Model file for the job. Use its own axes, mm. A direction names the side the tool comes from. Round coordinates to 2 decimals unless told otherwise and drop trailing zeros. Order: outer loops, then holes, each group sorted by start corner. A loop starts at its lowest first (then second) coordinate and runs counter-clockwise, first axis right, second up. Notation, with made-up numbers: (62.5, -0.5) - (95.5, -0.5) arc R16 ccw to (95.5, 17.5) - close; hole circle Ø3 at (58, 78). An arc over 180 degrees is marked (long way). Put each result on its own line as item: value. Start each with the question number.
Item 1: Mould opens along Z. For faces 4 (the face through (0, 0, -110)), 5 (the face through (23.846, -7.509, -102.395)), 6 (the face through (-17, -17, 65)) say: pulls with the +Z half, pulls with the -Z half, needs draft (parallel to the pull), parting line crosses it, or undercut.
Item 2: Pin check, flat tips, straight feed: pin 1 Ø8 at (x, z) = (-15, -51.5) entering from -Y; pin 2 Ø2.5 at (x, y) = (0, 17.5) entering from +Z; pin 3 Ø2.5 at (x, y) = (0, -17.5) entering from -Z. Stop position of each tip, or through.
Item 3: Probe probe 1 along Y at (x, z) = (0, -102.25); probe 2 along Z at (x, y) = (20, -5.5); probe 3 along X at (y, z) = (-17, -103). List the from-to ranges inside material, lowest first.
Item 4: Which spindle directions (+Z, -Z, +X, -X, +Y, -Y) get a long thin tool onto all of the face, cutting with end or side? Do faces 1 (the face through (22.4, 7.1, -13.9)), 2 (the face through (-1.08, -4.88, 112.96)), 3 (the face through (0, 0, 116)). Say none if no direction does.
Item 5: Saw through at B-B on x = 7.5. List the corners of the cut face in (y, z).
Item 6: Saw through at A-A on z = -40.5. List the corners of the cut face in (x, y).
```python
from build123d import *

# Parameters (mm, degrees)
SKETCH1_R                 = 23.5
BOSS_EXTRUDE1_DEPTH       = 110
SKETCH2_R                 = 5
BOSS_EXTRUDE2_DEPTH       = 6
SKETCH5_R                 = 25
BOSS_EXTRUDE5_DEPTH       = 45
BOSS_EXTRUDE6_START       = -15
SKETCH6_R                 = 25
BOSS_EXTRUDE6_DEPTH       = 15
M4X0_7_TAPPED_HOLE1_D     = 3.3
M4X0_7_TAPPED_HOLE1_DEPTH = 20
M4X0_7_TAPPED_HOLE1_TIP   = 0.991420021


with BuildPart() as part:
    # Sketch1 → Boss-Extrude1 (new, symmetric)
    with BuildSketch(Plane.XY):
        Circle(SKETCH1_R)
    extrude(amount=BOSS_EXTRUDE1_DEPTH, both=True)

    # Sketch2 → Boss-Extrude2 (add)
    with BuildSketch(Plane.XY.offset(110)):
        Circle(SKETCH2_R)
    extrude(amount=BOSS_EXTRUDE2_DEPTH)

    # Sketch5 → Boss-Extrude5 (add)
    with BuildSketch(Plane.XY.offset(110)):
        Circle(SKETCH5_R)
    extrude(amount=-BOSS_EXTRUDE5_DEPTH)

    # Sketch6 → Boss-Extrude6 (add)
    with BuildSketch(Plane(origin=(0, 0, -110), x_dir=(-1, 0, 0), z_dir=(0, 0, -1)).offset(BOSS_EXTRUDE6_START)):
        with Locations(Location((0, 0, 0), (0, 0, 180))):
            Circle(SKETCH6_R)
    extrude(amount=BOSS_EXTRUDE6_DEPTH)

    # M4x0.7 Tapped Hole1
    with Locations(Plane(origin=(0, 17.5, -110), x_dir=(-1, 0, 0), z_dir=(0, 0, -1))):
        with Locations((0, 0), (17.5, -17.5), (0, -35), (-17.5, -17.5)):
            Hole(M4X0_7_TAPPED_HOLE1_D / 2, depth=M4X0_7_TAPPED_HOLE1_DEPTH)
            with Locations((0, 0, -(M4X0_7_TAPPED_HOLE1_DEPTH + M4X0_7_TAPPED_HOLE1_TIP / 2))):  # 118° drill point
                Cone(0, M4X0_7_TAPPED_HOLE1_D / 2, M4X0_7_TAPPED_HOLE1_TIP, mode=Mode.SUBTRACT)


solid = part.part
```
Results found:
1. face 4: pulls with the -Z half
1. face 5: needs draft
1. face 6: undercut
2. pin 1: stops at y = -20.77
2. pin 2: stops at z = 110
2. pin 3: stops at z = -89.76
3. probe 1: y = -25 to -19.15, -15.85 to 15.85, 19.15 to 25
3. probe 2: z = -110 to 110
3. probe 3: x = -18.33 to -1.57, 1.57 to 18.33
4. face 1: none
4. face 2: +Z
4. face 3: +Z, +X, -X, +Y, -Y
5. outline: (-23.85, -110) - (23.85, -110) - (23.85, -95) - (22.27, -95) - (22.27, 65) - (23.85, 65) - (23.85, 110) - (-23.85, 110) - (-23.85, 65) - (-22.27, 65) - (-22.27, -95) - (-23.85, -95) - close
6. outline: circle Ø47 at (0, 0)
